Geometry: final body of the model. Coordinates: model frame, mm. Face numbers are marked on the shaded views. A direction names the side the tool comes from. Give positions to 0.01 mm unless a question says otherwise; leave off trailing zeros. Write each loop counter-clockwise with the first axis right and the second up, starting at its lowest first coordinate (ties: lowest second). Pieces come first, ordered by that corner, then holes. Notation, with made-up numbers: (8.25, -11) - (40.25, -11) arc R18 ccw to (40.25, 16) - close; hole circle Ø1 at (-14.75, 21). An arc over 180 degrees is marked (long way). Use CSV: the item, a comma, the result in double quotes. Start each with the question number.
(1) Section B-B on z = 9.75. Output: boundary loops of the cut face in (x, y), and give its area (3 significant figures).
(2) Line query: probe 1 along Y at (x, z) = (-2.5, 1.5); probe 2 along Y at (x, z) = (-2, 1); probe 3 along Z at (x, y) = (-3.5, 73). Output: solid intervals per line, ascending. Write a range as [from, to].
(3) Draft query along X for the marked faces 4, 5, 6 and 7. Return one class per face: released by +X, released by -X, zero draft, split by the parting line, or undercut.
(4) Reachability of the marked faces 1, 2 and 3 from +Z, -Z, +X, -X, +Y, -Y: full face, straight path, thin tool, end or side. Return the list, or none.
(5) Section C-C on x = 17.5. Output: boundary loops of the cut face in (y, z).
(6) First-contact query: pin 1 Ø4 at (y, z) = (77.5, 8) entering from -X; pin 2 Ø17 at (x, y) = (21, 53) entering from -Z; pin 3 Ø8 at (x, y) = (19.35, 50.41) entering from -Z; pin 4 Ø11.5 at (x, y) = (0.47, 63.02) entering from -Z. Flat tips, straight axial feed; report the tip coordinate or a pass-through.
(7) Section A-A on x = 1. Output: boundary loops of the cut face in (y, z), and give its area (3 significant figures).
(8) Section D-D on y = 70. Output: boundary loops of the cut face in (x, z).
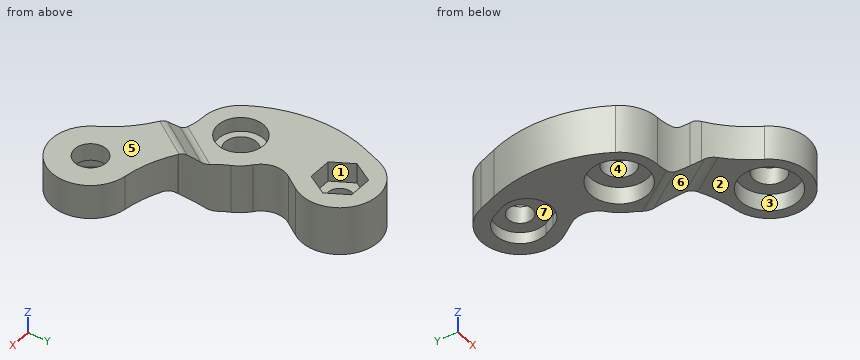
from build123d import *

# Parameters (mm, degrees)
SKETCH3_R               = 2.75
SKETCH3_R_2             = 2.1
BOSS_EXTRUDE2_DEPTH     = 11
CUT_EXTRUDE3_DEPTH      = 58.508197856
CUT_EXTRUDE3_DEPTH_BACK = 58.508197856
CUT_EXTRUDE5_DEPTH      = 91.859562292
CUT_EXTRUDE5_DEPTH_BACK = 3
SKETCH9_R               = 5
SKETCH10_R              = 5
CUT_EXTRUDE6_DEPTH      = 3
SKETCH11_R              = 4
CUT_EXTRUDE7_DEPTH      = 2.5
CUT_EXTRUDE8_DEPTH      = 2
CUT_EXTRUDE9_DEPTH      = 3.5


with BuildPart() as part:
    # Sketch3 → Boss-Extrude2 (new body)
    with BuildSketch(Plane.XY):
        with BuildLine():
            Line((11.81639044, 60.252883085), (11.728372068, 60.311638564))
            ThreePointArc((11.728372068, 60.311638564), (8.917204522, 62.7925154), (6.866230988, 65.931132995))
            ThreePointArc((6.866230988, 65.931132995), (6.025591445, 67.274340702), (4.901176311, 68.390840765))
            ThreePointArc((4.901176311, 68.390840765), (3.375934297, 70.989881123), (4.020351516, 73.93370524))
            Line((4.020351516, 73.93370524), (5.678869184, 76.41823992))
            ThreePointArc((5.678869184, 76.41823992), (3.137547336, 86.100651278), (-6.171856019, 82.420649156))
            Line((-6.171856019, 82.420649156), (-7.290261888, 79.347854286))
            ThreePointArc((-7.290261888, 79.347854286), (-8.557893098, 69.185727028), (-5.279809822, 59.483671095))
            ThreePointArc((-5.279809822, 59.483671095), (-2.848156457, 57.139360441), (0.414833066, 56.266646336))
            ThreePointArc((0.414833066, 56.266646336), (3.287818882, 55.822166382), (5.91364728, 54.574514525))
            Line((5.91364728, 54.574514525), (7.374782695, 53.599153256))
            ThreePointArc((7.374782695, 53.599153256), (10.815902262, 50.678650143), (13.499590609, 47.049812979))
            ThreePointArc((13.499590609, 47.049812979), (24.965953819, 46.665736496), (20.21385057, 57.108078892))
            ThreePointArc((20.21385057, 57.108078892), (15.833272198, 58.194897845), (11.81639044, 60.252883085))
        make_face()
        with Locations((19.351869275, 50.413343031)):
            Circle(SKETCH3_R, mode=Mode.SUBTRACT)
        with Locations((0.471910886, 63.016405008)):
            Circle(SKETCH3_R, mode=Mode.SUBTRACT)
        with Locations((0.114687614, 80.132534397)):
            Circle(SKETCH3_R_2, mode=Mode.SUBTRACT)
    extrude(amount=BOSS_EXTRUDE2_DEPTH)

    # Sketch8 → Cut-Extrude3 (cut, two sides: drawn at the far end of the back side and taken through both)
    with BuildSketch(Plane(origin=(31.465333136, 47.136495989, 0), x_dir=(0.8317162286287604, -0.5552009681507695, 0), z_dir=(0.5552009681507695, 0.8317162286287604, 0)).offset(-CUT_EXTRUDE3_DEPTH_BACK)):
        with BuildLine():
            Line((-28.1811996, -8.5), (-53.409946657, -8.5))
            Line((-53.409946657, -8.5), (-53.409946657, -11))
            Line((-53.409946657, -11), (-23.817856355, -11))
            ThreePointArc((-23.817856355, -11), (-24.442424101, -10.890774833), (-24.99285353, -10.576064729))
            Line((-24.99285353, -10.576064729), (-26.967564109, -8.937875854))
            ThreePointArc((-26.967564109, -8.937875854), (-27.536093723, -8.612816901), (-28.1811996, -8.5))
        make_face()
        with BuildLine():
            Line((-29.17758863, 0), (1.736877707, 0))
            Line((1.736877707, 0), (1.736877707, -5))
            Line((1.736877707, -5), (-21.22396203, -5))
            ThreePointArc((-21.22396203, -5), (-22.252174442, -4.820184962), (-23.158334542, -4.302084505))
            Line((-23.158334542, -4.302084505), (-27.702732311, -0.532123504))
            ThreePointArc((-27.702732311, -0.532123504), (-28.393631267, -0.137099418), (-29.17758863, 0))
        make_face()
    extrude(amount=CUT_EXTRUDE3_DEPTH + CUT_EXTRUDE3_DEPTH_BACK, mode=Mode.SUBTRACT)

    # Sketch9 → Cut-Extrude5 (cut, two sides: drawn at the far end of the back side and taken through both)
    with BuildSketch(Plane(origin=(0, 0, 5), x_dir=(-1, 0, 0), z_dir=(0, 0, -1)).offset(-CUT_EXTRUDE5_DEPTH_BACK)):
        with Locations(Location((-19.351869275, 50.413343031, 0), (0, 0, 180))):
            Circle(SKETCH9_R)
    extrude(amount=CUT_EXTRUDE5_DEPTH + CUT_EXTRUDE5_DEPTH_BACK, mode=Mode.SUBTRACT)

    # Sketch10 → Cut-Extrude6 (cut)
    with BuildSketch(Plane(origin=(0, 0, 0), x_dir=(-1, 0, 0), z_dir=(0, 0, -1))):
        with Locations((-0.471910886, 63.016405008)):
            Circle(SKETCH10_R)
    extrude(amount=-CUT_EXTRUDE6_DEPTH, mode=Mode.SUBTRACT)

    # Sketch11 → Cut-Extrude7 (cut)
    with BuildSketch(Plane.XY.offset(8.5)):
        with Locations((0.471910886, 63.016405008)):
            Circle(SKETCH11_R)
    extrude(amount=-CUT_EXTRUDE7_DEPTH, mode=Mode.SUBTRACT)

    # Sketch12 → Cut-Extrude8 (cut)
    with BuildSketch(Plane(origin=(0, 0, 0), x_dir=(-1, 0, 0), z_dir=(0, 0, -1))):
        with BuildLine():
            Line((3.691805092, 81.907531096), (4.579303441, 80.004284743))
            ThreePointArc((4.579303441, 80.004284743), (2.547807435, 74.422795339), (-3.03368197, 76.454291345))
            Line((-3.03368197, 76.454291345), (-3.92118032, 78.357537698))
            ThreePointArc((-3.92118032, 78.357537698), (-1.889684313, 83.939027102), (3.691805092, 81.907531096))
        make_face()
    extrude(amount=-CUT_EXTRUDE8_DEPTH, mode=Mode.SUBTRACT)

    # Sketch7 → Cut-Extrude9 (cut)
    with BuildSketch(Plane.XY.offset(8.5)):
        Polygon((2.16428107, 76.582534397), (4.213874525, 80.132534397), (2.16428107, 83.682534397), (-1.934905842, 83.682534397), (-3.984499297, 80.132534397), (-1.934905842, 76.582534397), align=None)
    extrude(amount=-CUT_EXTRUDE9_DEPTH, mode=Mode.SUBTRACT)


solid = part.part
Check values:
1,outline,"(5.4, 54.9) arc R10.06 cw to (5.91, 54.57) - (7.37, 53.6) arc R19.64 cw to (13.5, 47.05) arc R6.75 ccw (long way) to (20.21, 57.11) arc R19.64 cw to (11.82, 60.25) - (11.73, 60.31) arc R13.98 cw to (9.95, 61.72) - close; hole circle Ø5.5 at (19.35, 50.41)"
1,area,"187 mm²"
2,probe 1,"y = [56.96, 59], [67.04, 74.4], [83.42, 86.29]"
2,probe 2,"y = [56.74, 58.67], [67.36, 74.21], [83.76, 86.48]"
2,probe 3,"z = [0, 8.5]"
3,face 4,"undercut"
3,face 5,"zero draft"
3,face 6,"released by +X"
3,face 7,"undercut"
4,face 1,"+Z"
4,face 2,"-Z, +X, -Y"
4,face 3,"-Z"
5,outline,"(43.92, 5) - (45.77, 5) - (45.77, 8) - (48.38, 8) - (48.38, 11) - (43.92, 11) - close; (52.45, 8) - (55.06, 8) - (55.06, 5) - (57.65, 5) - (57.65, 11) - (52.45, 11) - close"
6,pin 1,"stops at x = -8.32"
6,pin 2,"stops at z = 5"
6,pin 3,"stops at z = 8"
6,pin 4,"stops at z = 0"
7,outline,"(56.24, 0) - (58.04, 0) - (58.04, 3) - (60.32, 3) - (60.32, 6) - (59.05, 6) - (59.05, 8.5) - (56.24, 8.5) - close; (65.72, 3) - (67.99, 3) - (67.99, 0) - (74.42, 0) - (74.42, 2) - (78.23, 2) - (78.23, 5) - (76.58, 5) - (76.58, 8.5) - (66.98, 8.5) - (66.98, 6) - (65.72, 6) - close; (82.04, 2) - (84.24, 2) - (84.24, 0) - (86.76, 0) - (86.76, 8.5) - (83.68, 8.5) - (83.68, 5) - (82.04, 5) - close"
7,area,"138 mm²"
8,outline,"(-8.63, 0) - (3.66, 0) - (3.66, 8.5) - (-8.63, 8.5) - close"
